For this review, use the dimensioned drawing (mm, ordinates from the lowest corner) and the shaded views. A direction names the side the tool comes from. Give positions to 0.01 mm unless a question says otherwise; leave off trailing zeros. Order: outer loops, then holes, each group sorted by start corner. A loop starts at its lowest first (then second) coordinate and runs counter-clockwise, first axis right, second up.
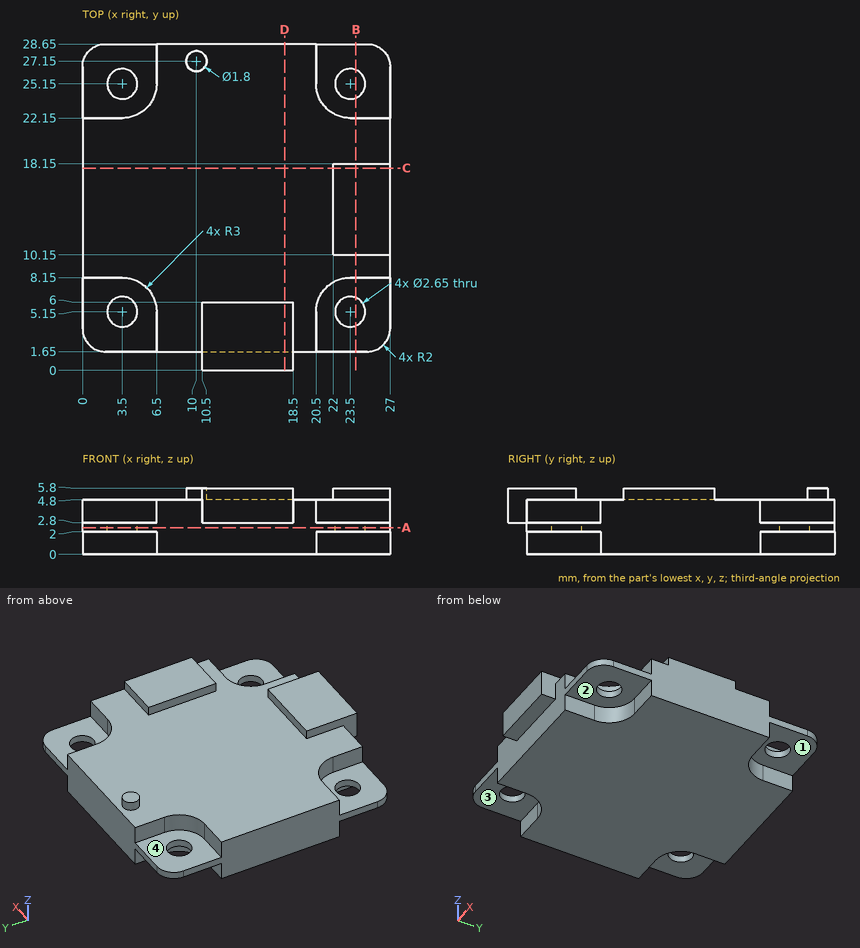
1. For pin 1 (0.6 mm diameter, centred on x = 25.5, z = 4, fed in from +Y); pin 2 (3 mm diameter, centred on x = 23, y = 25, fed in from +Z); pin 3 (1.6 mm diameter, centred on y = 27.5, z = 0.5, fed in from +X), all flat-tipped, find the tip position at first contact; note any pin that passes through.
Recorded:
pin 1: stops at y = 22.15
pin 2: stops at z = 2.8
pin 3: stops at x = 20.5
2. For line 1 along X through (y, z) = (25.15, 2.3) (3 decimals); line 2 along Y through (x, z) = (23.5, 2.5) (3 decimals); line 3 along Z through (x, y) = (21, 3.5), list the stretches that pass through material, from the lowest coordinate up.
Recorded:
line 1: x = 0 to 2.175, 4.825 to 22.175, 24.825 to 27
line 2: y = 1.65 to 3.825, 6.475 to 23.825, 26.475 to 28.65
line 3: z = 2 to 2.8
3. Take a section at C-C (y = 17.75). State the section outline as (x, z) points, then the cut area to 3 significant figures.
Recorded:
outline: (0, 0) - (27, 0) - (27, 5.8) - (22, 5.8) - (22, 4.8) - (0, 4.8) - close
area: 135 mm2
4. Take a section at A-A (z = 2.35). State the section outline as (x, y) points (3 decimals), then the cut area to 3 significant figures.
Recorded:
outline: (0, 3.65) arc R2 ccw to (2, 1.65) - (25, 1.65) arc R2 ccw to (27, 3.65) - (27, 26.65) arc R2 ccw to (25, 28.65) - (2, 28.65) arc R2 ccw to (0, 26.65) - close; hole circle Ø2.65 at (3.5, 5.15); hole circle Ø2.65 at (3.5, 25.15); hole circle Ø2.65 at (23.5, 5.15); hole circle Ø2.65 at (23.5, 25.15)
area: 704 mm2
5. Machinability: for the marked faces 1, 2, 3 and 4, which of the approach directions +Z, -Z, +X, -X, +Y, -Y give a long, thin tool a straight path to every point of the face, cutting with its end or side? Answer none if there is none.
Recorded:
face 1: -Z, +X, +Y
face 2: -Z, +X, -Y
face 3: -Z, -X, -Y
face 4: +Z, -X, +Y
6. Take a section at D-D (x = 17.75). State the section outline as (y, z) points, then the cut area to 3 significant figures.
Recorded:
outline: (0, 2.8) - (1.65, 2.8) - (1.65, 0) - (28.65, 0) - (28.65, 4.8) - (6, 4.8) - (6, 5.8) - (0, 5.8) - close
area: 139 mm2
7. Take a section at B-B (x = 24). State the section outline as (y, z) points, then the cut area to 3 significant figures.
Recorded:
outline: (1.65, 2) - (3.92, 2) - (3.92, 2.8) - (1.65, 2.8) - close; (6.38, 2) - (8.15, 2) - (8.15, 0) - (22.15, 0) - (22.15, 2) - (23.92, 2) - (23.92, 2.8) - (22.15, 2.8) - (22.15, 4.8) - (18.15, 4.8) - (18.15, 5.8) - (10.15, 5.8) - (10.15, 4.8) - (8.15, 4.8) - (8.15, 2.8) - (6.38, 2.8) - close; (26.38, 2) - (28.65, 2) - (28.65, 2.8) - (26.38, 2.8) - close
area: 81.7 mm2
